Design review of the part built by this model. Coordinates are the model's own, in mm. Coordinates: 2 decimals unless noted, no trailing zeros. Write each loop counter-clockwise with the first axis right and the second up, starting at its lowest first coordinate (ties: lowest second). Pieces come first, ordered by that corner, then holes. Notation, with made-up numbers: (28.25, -20) - (59.25, -20) arc R14 cw to (59.25, 2) - close; hole circle Ø5 at (-13.5, 17.5). An arc over 180 degrees is marked (long way). Answer as CSV lines item,"result". Start each with the question number.
Q1. We need section C-C (x = 108). Write out the cut boundary in (y, z).
Q2. We need section A-A (x = 191.5). Write out the cut boundary in (y, z), plus the area to 3 significant figures.
Q3. Clearance check with flat-ended pins moving along their axes: pin 1 (6 mm diameter, centred on x = -22.5, y = 0, fed in from -Z); pin 2 (1.2 mm diameter, centred on y = 2, z = 2, fed in from +X). State where each tip first meets the part, or that it passes through.
Q4. For line 1 along Y through (x, z) = (220, 1.9); line 2 along Y through (x, z) = (0.5, 0.65); line 3 along Y through (x, z) = (47, 2.15), list the stretches that pass through material, from the lowest coordinate up. Write a range as [from, to].
Q5. We need section B-B (z = 1.8). State how many separate pieces and enclosed holes the cut face has, plus the area to 3 significant figures.
from build123d import *

# Parameters (mm, degrees)
SKETCH_1_R          = 5.2
SKETCH_1_R_2        = 9.7
EXTRUDE_1_DEPTH     = 4
SKETCH_2_R          = 2
CUT_EXTRUDE_1_DEPTH = 10
SKETCH_3_R          = 5
CUT_EXTRUDE_2_DEPTH = 10


with BuildPart() as part:
    # 草图1 → 凸台-拉伸1 (new body)
    with BuildSketch(Plane.XY):
        with BuildLine():
            Line((250, 19.7), (0, 19.7))
            Line((0, 19.7), (-45, 15.2))
            ThreePointArc((-45, 15.2), (-60.2, 0), (-45, -15.2))
            Line((-45, -15.2), (0, -19.7))
            Line((0, -19.7), (250, -19.7))
            ThreePointArc((250, -19.7), (269.7, 0), (250, 19.7))
        make_face()
        Circle(SKETCH_1_R, mode=Mode.SUBTRACT)
        with Locations((250, 0)):
            Circle(SKETCH_1_R_2, mode=Mode.SUBTRACT)
        with Locations((-45, 0)):
            Circle(SKETCH_1_R, mode=Mode.SUBTRACT)
    extrude(amount=EXTRUDE_1_DEPTH)

    # 草图2 → 切除-拉伸1 (cut)
    with BuildSketch(Plane.XY.offset(4)):
        with Locations((25, 15)):
            Circle(SKETCH_2_R)
        with Locations((90, 15)):
            Circle(SKETCH_2_R)
        with Locations((155, 15)):
            Circle(SKETCH_2_R)
        with Locations((220, 15)):
            Circle(SKETCH_2_R)
        with Locations((90, -15)):
            Circle(SKETCH_2_R)
        with Locations((155, -15)):
            Circle(SKETCH_2_R)
        with Locations((220, -15)):
            Circle(SKETCH_2_R)
        with Locations((25, -15)):
            Circle(SKETCH_2_R)
    extrude(amount=-CUT_EXTRUDE_1_DEPTH, mode=Mode.SUBTRACT)

    # 草图3 → 切除-拉伸2 (cut)
    with BuildSketch(Plane.XY.offset(4)):
        with Locations((-22.5, 0)):
            Circle(SKETCH_3_R)
        with BuildLine():
            Line((32, 8), (32, -8))
            Line((32, -8), (88.462542093, -8))
            Line((88.462542093, -8), (114.86138476, 4.184081231))
            ThreePointArc((114.86138476, 4.184081231), (115.976706085, 6.429046887), (114.023268405, 8))
            Line((114.023268405, 8), (32, 8))
        make_face()
        with BuildLine():
            Line((156.537457907, 8), (213, 8))
            Line((213, 8), (213, -8))
            Line((213, -8), (130.976731595, -8))
            ThreePointArc((130.976731595, -8), (129.023293915, -6.429046887), (130.13861524, -4.184081231))
            Line((130.13861524, -4.184081231), (156.537457907, 8))
        make_face()
    extrude(amount=-CUT_EXTRUDE_2_DEPTH, mode=Mode.SUBTRACT)


solid = part.part
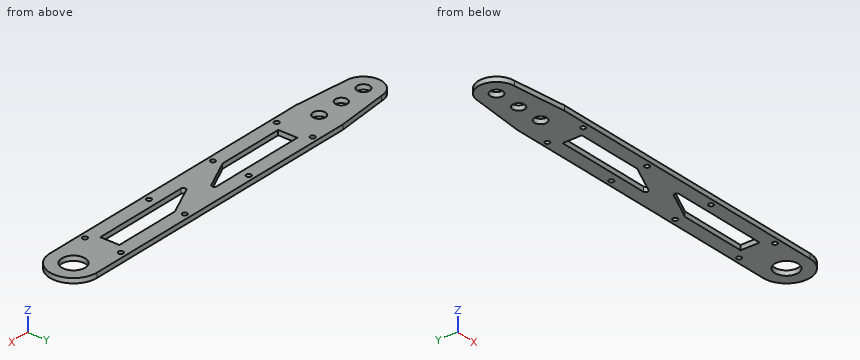
Results list:
1,outline,"(-19.7, 0) - (1.02, 0) - (1.02, 4) - (-19.7, 4) - close; (8, 0) - (19.7, 0) - (19.7, 4) - (8, 4) - close"
2,outline,"(-19.7, 0) - (-8, 0) - (-8, 4) - (-19.7, 4) - close; (8, 0) - (19.7, 0) - (19.7, 4) - (8, 4) - close"
2,area,"93.6 mm2"
3,pin 1,"passes through"
3,pin 2,"stops at x = 269.65"
4,line 1,"y = [-19.7, -17], [-13, 13], [17, 19.7]"
4,line 2,"y = [-19.7, -5.18], [5.18, 19.7]"
4,line 3,"y = [-19.7, -8], [8, 19.7]"
5,separate pieces,"1"
5,enclosed holes,"14"
5,area,"9,410 mm2"
